Verification items for the finished model (mm, model axes). Face numbers are marked on the shaded views. A direction names the side the tool comes from. Coordinates: 2 decimals unless noted, no trailing zeros. Order: outer loops, then holes, each group sorted by start corner. A loop starts at its lowest first (then second) coordinate and runs counter-clockwise, first axis right, second up. Notation, with made-up numbers: M 7.5,45 L 15.5,45 A24 ccw 15.5,79 Z; hole C 54,-29 d2. An arc over 180 degrees is marked long. Return JSON: item names as keys, results as strings. Group by question number.
Q1. Access from +Z, -Z, +X, -X, +Y, -Y to the whole of each face (thin tool, end or side, straight path). Record for the marked faces 1 and 2.
Q2. Thickness scan on probe 1 along Y at (x, z) = (150, 5.25); probe 2 along Y at (x, z) = (125.5, 3); probe 3 along X at (y, z) = (-4.5, 13). Record the ranges inside material, lowest first.
Q3. Section check C-C, the plane z = 7.5. Count the separate pieces of the cut face and the enclosed holes in it, then the cut area to 3 significant figures.
Q4. Section check A-A, the plane y = 39. Enter the section's corners in (x, z), then the cut area to 3 significant figures.
Q5. Section check B-B, the plane x = 193. Enter the section's corners in (y, z), then the cut area to 3 significant figures.
Q6. Go/stop test with flat-tipped pins: pin 1 Ø2 at (y, z) = (20, 13) entering from -X; pin 2 Ø5 at (x, y) = (189, -36.5) entering from +Z; pin 3 Ø12 at (x, z) = (159.5, 7) entering from +Y; pin 4 Ø10 at (y, z) = (-16.5, 4.5) entering from -X. Record where each tip stops, or that it passes through.
Q7. Mould release check, pull along Y, two halves, no side actions. Record for the marked faces 3, 4, 5 and 6: pulls with the +Y half, pulls with the -Y half, needs draft (parallel to the pull), parting line crosses it, or undercut.
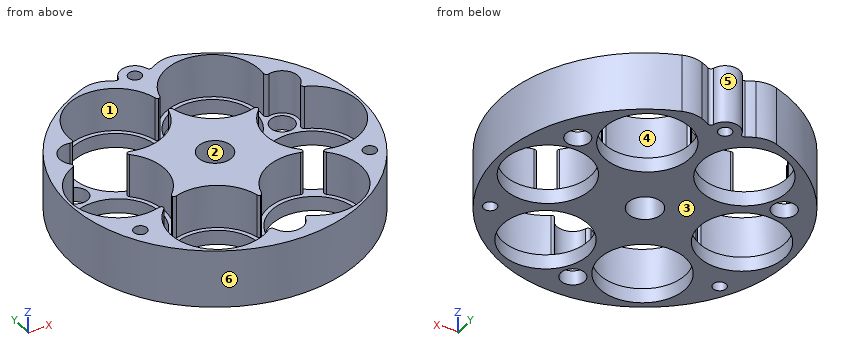
from build123d import *

# Parameters (mm, degrees)
EXTRUDE_1_DEPTH               = 20
CUT_EXTRUDE_1_DEPTH           = 15
EXTRUDE_2_DEPTH               = 15
HOLE_WIZARD_11_5_11_5_1_D     = 11.5
HOLE_WIZARD_11_5_11_5_1_DEPTH = 20
HOLE_WIZARD_4_5_4_5_1_D       = 4.5
HOLE_WIZARD_4_5_4_5_1_DEPTH   = 20
HOLE_WIZARD_8_2_8_2_1_D       = 8.2
HOLE_WIZARD_8_2_8_2_1_DEPTH   = 20
HOLE_WIZARD_M27_1_D           = 29.5
HOLE_WIZARD_M27_1_DEPTH       = 20
FILLET_1_R                    = 10


with BuildPart() as part:
    # 草图1 → 凸台-拉伸1 (new body)
    with BuildSketch(Plane(origin=(0, 0, 0), x_dir=(-1, 0, 0), z_dir=(0, 0, -1))):
        with BuildLine():
            ThreePointArc((-163.044825793, 48.268338691), (-150.013943269, -49.999998056), (-136.9282555, 48.261055684))
            ThreePointArc((-136.9282555, 48.261055684), (-140.436485638, 47.315672166), (-143.715786974, 45.751187764))
            ThreePointArc((-143.715786974, 45.751187764), (-144.598832064, 45.682763471), (-145.189860946, 46.34241139))
            ThreePointArc((-145.189860946, 46.34241139), (-149.9980945, 49.999993293), (-154.818283841, 46.35818193))
            ThreePointArc((-154.818283841, 46.35818193), (-155.409600478, 45.701218741), (-156.290828184, 45.76972954))
            ThreePointArc((-156.290828184, 45.76972954), (-159.554442065, 47.325525228), (-163.044825793, 48.268338691))
        make_face()
    extrude(amount=-EXTRUDE_1_DEPTH)

    # 草图2 → 切除-拉伸1 (cut)
    with BuildSketch(Plane.XY.offset(20)):
        with BuildLine():
            ThreePointArc((182.530473967, 26.658794029), (169.344288449, 44.464391856), (150.792813346, 32.350037808))
            ThreePointArc((150.792813346, 32.350037808), (150.506114031, 31.856143154), (149.995856029, 31.599695892))
            ThreePointArc((149.995856029, 31.599695892), (149.485428939, 31.855806439), (149.198403823, 32.349511827))
            ThreePointArc((149.198403823, 32.349511827), (130.657581348, 44.454967541), (117.460046658, 26.674944082))
            ThreePointArc((117.460046658, 26.674944082), (117.13046307, 25.810318318), (116.2327011, 25.586205625))
            ThreePointArc((116.2327011, 25.586205625), (110.175484721, 22.978350815), (110.975201971, 16.432265779))
            ThreePointArc((110.975201971, 16.432265779), (111.233397945, 15.540844642), (110.647570153, 14.821051199))
            ThreePointArc((110.647570153, 14.821051199), (101.822353243, -5.506280624), (121.597754537, -15.507199392))
            ThreePointArc((121.597754537, -15.507199392), (122.167866534, -15.507879551), (122.644955628, -15.819991947))
            ThreePointArc((122.644955628, -15.819991947), (122.677083904, -16.389198347), (122.392942981, -16.883457477))
            ThreePointArc((122.392942981, -16.883457477), (121.168678782, -38.996245439), (143.168797451, -41.539666912))
            ThreePointArc((143.168797451, -41.539666912), (144.082377122, -41.39278179), (144.725345392, -42.058210116))
            ThreePointArc((144.725345392, -42.058210116), (150.012422097, -45.999985972), (155.281639409, -42.034367999))
            ThreePointArc((155.281639409, -42.034367999), (155.924534771, -41.365053158), (156.840808075, -41.512498187))
            ThreePointArc((156.840808075, -41.512498187), (178.860797944, -38.987667291), (177.623107818, -16.85798478))
            ThreePointArc((177.623107818, -16.85798478), (177.338551357, -16.365073167), (177.369025987, -15.796737408))
            ThreePointArc((177.369025987, -15.796737408), (177.845776872, -15.485863106), (178.414928942, -15.485464907))
            ThreePointArc((178.414928942, -15.485464907), (198.1856076, -5.497255844), (189.390008085, 14.832069871))
            ThreePointArc((189.390008085, 14.832069871), (188.806012002, 15.549810513), (189.060805702, 16.439351532))
            ThreePointArc((189.060805702, 16.439351532), (189.830945377, 22.988982198), (183.762010815, 25.569449262))
            ThreePointArc((183.762010815, 25.569449262), (182.860919479, 25.791555557), (182.530473967, 26.658794029))
        make_face()
    extrude(amount=-CUT_EXTRUDE_1_DEPTH, mode=Mode.SUBTRACT)

    # 草图3 → 凸台-拉伸2 (add)
    with BuildSketch(Plane.XY.offset(5)):
        with BuildLine():
            ThreePointArc((150.806742296, -24.817251573), (150.522146149, -25.310140695), (150.014715092, -25.56791652))
            ThreePointArc((150.014715092, -25.56791652), (149.507114069, -25.310475545), (149.222192785, -24.817774301))
            ThreePointArc((149.222192785, -24.817774301), (141.584673617, -14.598117133), (128.913467977, -13.110286731))
            ThreePointArc((128.913467977, -13.110286731), (128.345273464, -13.110918369), (127.868454338, -12.801905545))
            ThreePointArc((127.868454338, -12.801905545), (127.838876563, -12.234481049), (128.123196321, -11.742538289))
            ThreePointArc((128.123196321, -11.742538289), (133.162564653, -0.011170953), (128.107804336, 11.71357258))
            ThreePointArc((128.107804336, 11.71357258), (127.823073861, 12.2041736), (127.851011875, 12.770724808))
            ThreePointArc((127.851011875, 12.770724808), (128.32748764, 13.078509879), (128.894726547, 13.077600818))
            ThreePointArc((128.894726547, 13.077600818), (141.579615252, 14.573425047), (149.210722651, 24.815987784))
            ThreePointArc((149.210722651, 24.815987784), (149.493229963, 25.307871928), (149.997846175, 25.566952748))
            ThreePointArc((149.997846175, 25.566952748), (150.502633213, 25.30820492), (150.785465, 24.816507277))
            ThreePointArc((150.785465, 24.816507277), (158.418767714, 14.58161384), (171.099107848, 13.088520381))
            ThreePointArc((171.099107848, 13.088520381), (171.667301632, 13.089152517), (172.144120652, 12.78014087))
            ThreePointArc((172.144120652, 12.78014087), (172.173697461, 12.212717053), (171.889377635, 11.720775173))
            ThreePointArc((171.889377635, 11.720775173), (166.85, -5.6959e-05), (171.889460311, -11.720853545))
            ThreePointArc((171.889460311, -11.720853545), (172.174016773, -12.213765158), (172.143542142, -12.782100917))
            ThreePointArc((172.143542142, -12.782100917), (171.666791258, -13.092975219), (171.097639187, -13.093373418))
            ThreePointArc((171.097639187, -13.093373418), (158.432956354, -14.595191678), (150.806742296, -24.817251573))
        make_face()
    extrude(amount=EXTRUDE_2_DEPTH)

    # Ø11.5 (11.5) 直径孔1
    with Locations(Plane(origin=(0, 0, 0), x_dir=(-1, 0, 0), z_dir=(0, 0, -1))):
        with Locations((-150, 0)):
            Hole(HOLE_WIZARD_11_5_11_5_1_D / 2, depth=HOLE_WIZARD_11_5_11_5_1_DEPTH)

    # Ø4.5 (4.5) 直径孔1
    with Locations(Plane(origin=(0, 0, 0), x_dir=(-1, 0, 0), z_dir=(0, 0, -1))):
        with Locations((-150.006284065, 45), (-111.025714797, -22.516326479), (-188.986853332, -22.516326479)):
            Hole(HOLE_WIZARD_4_5_4_5_1_D / 2, depth=HOLE_WIZARD_4_5_4_5_1_DEPTH)

    # Ø8.2 (8.2) 直径孔1
    with Locations(Plane(origin=(0, 0, 0), x_dir=(-1, 0, 0), z_dir=(0, 0, -1))):
        with Locations((-150, -40.5), (-114.944823341, 20.23911568), (-185.074028853, 20.228231361)):
            Hole(HOLE_WIZARD_8_2_8_2_1_D / 2, depth=HOLE_WIZARD_8_2_8_2_1_DEPTH)

    # M27 间隙孔1
    with Locations(Plane(origin=(0, 0, 0), x_dir=(-1, 0, 0), z_dir=(0, 0, -1))):
        with Locations((-183, 0), (-166.51256813, -28.578838325), (-133.518852195, -28.589722645), (-166.493715935, 28.567954005), (-117.01256813, -0.021768639), (-133.5, 28.557069686)):
            Hole(HOLE_WIZARD_M27_1_D / 2, depth=HOLE_WIZARD_M27_1_DEPTH)

    # 圆角1
    fillet_1_edges = [part.edges().sort_by_distance(p)[0] for p in [
        (136.9282555, 48.261055684, 10),
        (163.044825793, 48.268338691, 10),
    ]]
    fillet(fillet_1_edges, radius=FILLET_1_R)


solid = part.part
Numbers:
{
 "1": {"face 1": "+Z", "face 2": "+Z, -Z"},
 "2": {"probe 1": "y = -50 to -46, -25.57 to -5.75, 5.75 to 25.57, 31.6 to 42.75, 47.25 to 50", "probe 2": "y = -43.59 to -40.97, -16.21 to -12.09, 12.04 to 16.17, 40.95 to 43.59", "probe 3": "x = 100.2 to 101.5, 132.53 to 146.42, 153.58 to 167.49, 198.51 to 199.8"},
 "3": {"separate pieces": "2", "enclosed holes": "5", "area": "2,430 mm2"},
 "4": {"outline": "M 118.71,0 L 123.08,0 L 123.08,5 L 121.18,5 L 121.18,20 L 118.71,20 Z; M 143.92,0 L 156.07,0 L 156.07,5 L 154.17,5 L 154.17,20 L 145.82,20 L 145.82,5 L 143.92,5 Z; M 176.92,0 L 181.29,0 L 181.29,20 L 178.82,20 L 178.82,5 L 176.92,5 Z", "area": "304 mm2"},
 "5": {"outline": "M -25.51,0 L -10.84,0 L -10.84,5 L -12.68,5 L -12.68,20 L -25.51,20 Z; M 10.84,0 L 25.51,0 L 25.51,20 L 12.68,20 L 12.68,5 L 10.84,5 Z", "area": "532 mm2"},
 "6": {"pin 1": "stops at x = 103.75", "pin 2": "passes through", "pin 3": "stops at y = 48.58", "pin 4": "stops at x = 101.34"},
 "7": {"face 3": "needs draft", "face 4": "undercut", "face 5": "pulls with the +Y half", "face 6": "parting line crosses it"}
}
